Input: dimensioned drawing with shaded views. Units: mm. Origin: part minimum x, y, z. A direction names the side the tool comes from. Round coordinates to 2 decimals unless told otherwise and drop trailing zeros. Loops run counter-clockwise (first coordinate to the right, second up) from the corner with the lowest first, then second, coordinate; pieces in that order, holes last. Notation, with made-up numbers: M 18.25,75.5 L 30.25,75.5 A15 cw 30.25,90.5 Z; hole C 4,13.5 d6. An arc over 180 degrees is marked long. Return JSON: item names as keys, results as strings.
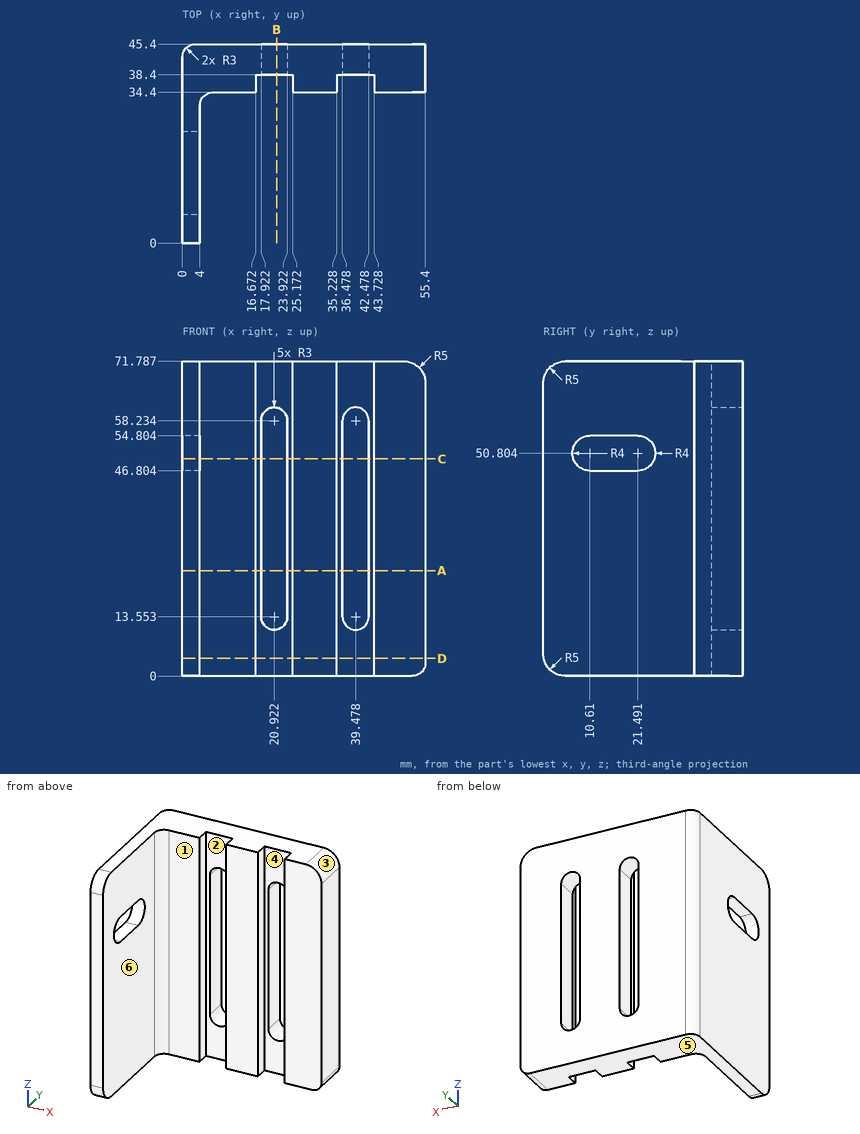
Q1. Reachability of the marked faces 4, 5 and 6 from +Z, -Z, +X, -X, +Y, -Y: full face, straight path, thin tool, end or side. Return the list, or none.
Determined:
{"face 4": "+Z, -Z, -Y", "face 5": "-Z, +X, -X, +Y, -Y", "face 6": "+Z, -Z, +X, -Y"}
Q2. Material intervals for L1, parallel to X at y = 41.5, z = 37; L2, parallel to X at y = 43.5, z = 33; L3, parallel to X at y = 29, z = 20, sorted ascending.
Determined:
{"L1": "x = 0 to 17.92, 23.92 to 36.48, 42.48 to 55.4", "L2": "x = 0.21 to 17.92, 23.92 to 36.48, 42.48 to 55.4", "L3": "x = 0 to 4"}
Q3. Section query C-C (z = 49.5). Output: boundary loops of the cut face in (x, y), plus the area to 3 significant figures.
Determined:
{"outline": "M 0,0 L 4,0 L 4,6.83 L 0,6.83 Z; M 0,25.27 L 4,25.27 L 4,31.4 A3 cw 7,34.4 L 16.67,34.4 L 16.67,38.4 L 17.92,38.4 L 17.92,45.4 L 3,45.4 A3 ccw 0,42.4 Z; M 23.92,38.4 L 25.17,38.4 L 25.17,34.4 L 35.23,34.4 L 35.23,38.4 L 36.48,38.4 L 36.48,45.4 L 23.92,45.4 Z; M 42.48,38.4 L 43.73,38.4 L 43.73,34.4 L 55.4,34.4 L 55.4,45.4 L 42.48,45.4 Z", "area": "521 mm^2"}
Q4. Section query A-A (z = 24). Output: boundary loops of the cut face in (x, y).
Determined:
{"outline": "M 0,0 L 4,0 L 4,31.4 A3 cw 7,34.4 L 16.67,34.4 L 16.67,38.4 L 17.92,38.4 L 17.92,45.4 L 3,45.4 A3 ccw 0,42.4 Z; M 23.92,38.4 L 25.17,38.4 L 25.17,34.4 L 35.23,34.4 L 35.23,38.4 L 36.48,38.4 L 36.48,45.4 L 23.92,45.4 Z; M 42.48,38.4 L 43.73,38.4 L 43.73,34.4 L 55.4,34.4 L 55.4,45.4 L 42.48,45.4 Z"}
Q5. Pin query (flat end, axial travel): pin 1 (6 mm diameter, centred on y = 5, z = 48.5, fed in from +X); pin 2 (7 mm diameter, centred on x = 21.5, z = 31, fed in from -Y); pin 3 (5 mm diameter, centred on x = 13.5, z = 49.5, fed in from -Y). Return the tip coordinate at first contact, or that it passes through.
Determined:
{"pin 1": "stops at x = 4", "pin 2": "stops at y = 38.4", "pin 3": "stops at y = 34.4"}
Q6. Pull-direction query (X, two-part tool) for the marked faces 1, 2 and 3; classes: pulls with the +X half, pulls with the -X half, needs draft (parallel to the pull), parting line crosses it, or undercut.
Determined:
{"face 1": "needs draft", "face 2": "undercut", "face 3": "pulls with the +X half"}
Q7. Section query B-B (x = 21.5). Output: boundary loops of the cut face in (y, z).
Determined:
{"outline": "M 38.4,0 L 45.4,0 L 45.4,10.61 L 38.4,10.61 Z; M 38.4,61.18 L 45.4,61.18 L 45.4,71.79 L 38.4,71.79 Z"}
Q8. Section query D-D (z = 4). Output: boundary loops of the cut face in (x, y).
Determined:
{"outline": "M 0,0.1 L 4,0.1 L 4,31.4 A3 cw 7,34.4 L 16.67,34.4 L 16.67,38.4 L 25.17,38.4 L 25.17,34.4 L 35.23,34.4 L 35.23,38.4 L 43.73,38.4 L 43.73,34.4 L 55.4,34.4 L 55.4,45.4 L 3,45.4 A3 ccw 0,42.4 Z"}
